The listing builds one solid part. Answer for the finished solid, in the listing's coordinates (mm). Give positions to 0.01 mm unless a question says otherwise; leave off trailing zeros. Loops run counter-clockwise (first coordinate to the right, second up) from the corner with the lowest first, then second, coordinate; pieces in that order, holes last. Notation, with made-up numbers: M 30,34.5 L 44,34.5 A27 cw 44,67.5 Z; hole C 74,70.25 d6. An arc over 180 degrees is marked long. Return JSON: item names as keys, results as strings.
from build123d import *

# Parameters (mm, degrees)
F0_W     = 238.125
F0_H     = 168.275
F1_DEPTH = 6.35
F3_DEPTH = 25.4
F5_DEPTH = 25.4
F6_R     = 5.08


with BuildPart() as f1:
    # F0 (on Top) → F1 (new body)
    with BuildSketch(Plane.XY):
        Rectangle(F0_W, F0_H)
    extrude(amount=F1_DEPTH)

    # F2 (on face) → F3 (cut)
    with BuildSketch(Plane.XY.offset(6.35)):
        Polygon((-35.7505, -1.0795), (-80.9625, 44.1325), (-80.9625, -46.0375), (72.359927, -46.0375), (72.359927, -1.0795), (59.11182, -14.327607), (27.321713, 17.4625), (-4.468393, -14.327607), (-35.7505, 16.9545), align=None)
    extrude(amount=-F3_DEPTH, mode=Mode.SUBTRACT)

    # F4 (on face) → F5 (cut)
    with BuildSketch(Plane.XY.offset(6.35)):
        with BuildLine():
            ThreePointArc((-35.676324, 18.676375), (-36.534425, 18.847062), (-37.0205, 18.119599))
            Line((-37.0205, 18.119599), (-37.0205, 3.887503))
            ThreePointArc((-37.0205, 3.887503), (-37.506575, 3.16004), (-38.364676, 3.330727))
            Line((-38.364676, 3.330727), (-80.888324, 45.854375))
            ThreePointArc((-80.888324, 45.854375), (-81.746425, 46.025062), (-82.2325, 45.297599))
            Line((-82.2325, 45.297599), (-82.2325, -46.5201))
            ThreePointArc((-82.2325, -46.5201), (-82.001876, -47.076876), (-81.4451, -47.3075))
            Line((-81.4451, -47.3075), (72.842527, -47.3075))
            ThreePointArc((72.842527, -47.3075), (73.399303, -47.076876), (73.629927, -46.5201))
            Line((73.629927, -46.5201), (73.629927, 0.085599))
            ThreePointArc((73.629927, 0.085599), (73.143852, 0.813062), (72.285751, 0.642375))
            Line((72.285751, 0.642375), (59.668596, -11.97478))
            ThreePointArc((59.668596, -11.97478), (59.11182, -12.205404), (58.555044, -11.97478))
            Line((58.555044, -11.97478), (27.878489, 18.701775))
            ThreePointArc((27.878489, 18.701775), (27.321713, 18.932399), (26.764937, 18.701775))
            Line((26.764937, 18.701775), (-3.911617, -11.97478))
            ThreePointArc((-3.911617, -11.97478), (-4.468393, -12.205404), (-5.025169, -11.97478))
            Line((-5.025169, -11.97478), (-35.676324, 18.676375))
        make_face()
    extrude(amount=-F5_DEPTH, mode=Mode.SUBTRACT)

    # F6
    f6_edges = [f1.edges().sort_by_distance(p)[0] for p in [
        (119.0625, 84.1375, 3.175),
        (119.0625, -84.1375, 3.175),
        (-119.0625, 84.1375, 3.175),
        (-119.0625, -84.1375, 3.175),
    ]]
    fillet(f6_edges, radius=F6_R)


solid = f1.part
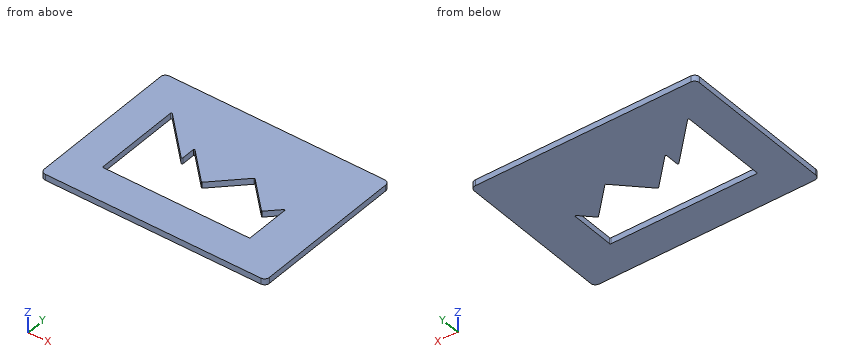
(1) The part is cut by section A-A (y = -36). Determine the outline of the cut face in (x, z).
Values follow:
{"outline": "M -119.06,0 L -82.23,0 L -82.23,6.35 L -119.06,6.35 Z; M 73.63,0 L 119.06,0 L 119.06,6.35 L 73.63,6.35 Z"}
(2) The part is cut by section B-B (z = 1.5). Determine the outline of the cut face in (x, y) (1 decimal).
Values follow:
{"outline": "M -119.1,-79.1 A5.1 ccw -114,-84.1 L 114,-84.1 A5.1 ccw 119.1,-79.1 L 119.1,79.1 A5.1 ccw 114,84.1 L -114,84.1 A5.1 ccw -119.1,79.1 Z; hole M -82.2,-46.5 A0.8 ccw -81.4,-47.3 L 72.8,-47.3 A0.8 ccw 73.6,-46.5 L 73.6,0.1 A0.8 ccw 72.3,0.6 L 59.7,-12 A0.8 cw 58.6,-12 L 27.9,18.7 A0.8 ccw 26.8,18.7 L -3.9,-12 A0.8 cw -5,-12 L -35.7,18.7 A0.8 ccw -37,18.1 L -37,3.9 A0.8 cw -38.4,3.3 L -80.9,45.9 A0.8 ccw -82.2,45.3 Z"}
(3) The part is cut by section D-D (y = 8). Determine the outline of the cut face in (x, z), and give its area (3 significant figures).
Values follow:
{"outline": "M -119.06,0 L -82.23,0 L -82.23,6.35 L -119.06,6.35 Z; M -43.03,0 L -37.02,0 L -37.02,6.35 L -43.03,6.35 Z; M -25,0 L 16.06,0 L 16.06,6.35 L -25,6.35 Z; M 38.58,0 L 119.06,0 L 119.06,6.35 L 38.58,6.35 Z", "area": "1,040 mm²"}
(4) Straight lines are drawn through the part: line 1 along X through (y, z) = (-35.5, 3); line 2 along X through (y, z) = (9, 2.25); line 3 along X through (y, z) = (4, 4). For each, find the intervals that lie inside material, in ascending order.
Values follow:
{"line 1": "-119.06 to -82.23, 73.63 to 119.06", "line 2": "-119.06 to -82.23, -44.03 to -37.02, -26 to 17.06, 37.58 to 119.06", "line 3": "-119.06 to -82.23, -39.03 to -37.02, -21 to 12.06, 42.58 to 119.06"}
(5) The part is cut by section C-C (x = 54). Determine the outline of the cut face in (y, z), and give its area (3 significant figures).
Values follow:
{"outline": "M -84.14,0 L -47.31,0 L -47.31,6.35 L -84.14,6.35 Z; M -7.42,0 L 84.14,0 L 84.14,6.35 L -7.42,6.35 Z", "area": "815 mm²"}
